For this review, take the finished solid that the model builds, in its own axes (mm). A direction names the side the tool comes from. Coordinates: 2 decimals unless noted, no trailing zeros. Order: outer loops, then holes, each group sorted by start corner. A loop starts at its lowest first (then second) coordinate and runs counter-clockwise, first axis right, second up. Notation, with made-up numbers: (-19, 10) -> (27, 10) arc R14 cw to (27, 28) -> close; hole circle Ø10 at (-24, -13). An arc over 180 degrees is marked (long way). Return JSON: item names as keys, results as strings. Group by question number.
Item 1: For line 1 along Y through (x, z) = (-13, 1); line 2 along Z through (x, y) = (29.5, 35); line 3 along X through (y, z) = (-1, 6), list the stretches that pass through material, from the lowest coordinate up.
Item 2: Take a section at A-A (y = 5). Write out the cut boundary in (x, z).
Item 3: Insertion check: pin 1 (12 mm diameter, centred on x = 0.5, y = 10.5, fed in from -Z); pin 2 (3 mm diameter, centred on x = 31.5, y = 80.5, fed in from +Z); pin 3 (3.5 mm diameter, centred on x = -36.93, y = 56.31, fed in from -Z); pin 4 (12 mm diameter, centred on y = -19.5, z = 9.5, fed in from -X). Each pin has a flat end and moves straight along its axis. Give the tip position at first contact, or say it passes through.
Item 4: Draft analysis for pull direction Z (two halves, no side actions). For faces 1 (the flat face through (0.57, -7.61, 11.68)), 2 (the flat face through (-10, -10, 4)), 3 (the cylindrical face through (0.567, -19.206, 5.344)), 4 (the cylindrical face through (-20.316, -19.206, 5.344)), state which applies: +Z half, -Z half, draft (parallel to the pull), parting line (faces both ways), or undercut.
Item 5: Take a section at B-B (x = 12.5). Write out the cut boundary in (y, z), then the cut area to 3 significant figures.
Item 6: Take a section at C-C (x = -6). Write out the cut boundary in (y, z).
Item 7: Take a section at D-D (z = -2.5). Write out the cut boundary in (x, y), then the cut area to 3 significant figures.
Item 8: Machinability: for faces 5 (the flat face through (10, -10, 4)), 6 (the flat face through (25, -16, 4)), 7 (the flat face through (20.183, -8.199, -3.475)), 8 (the flat face through (-20.316, -8.199, -3.475)), which of the approach directions +Z, -Z, +X, -X, +Y, -Y give a long, thin tool a straight path to every point of the face, cutting with its end or side? Answer none if there is none.
```python
from build123d import *

# Parameters (mm, degrees)
SKETCH_1_R                  = 2
SKETCH_1_R_2                = 23
EXTRUDE_1_DEPTH             = 8
SKETCH_2_R                  = 2.5
EXTRUDE_2_DEPTH             = 9.5
EXTRUDE_START               = -9.5
SKETCH_4_R                  = 2.5
EXTRUDE_4_DEPTH             = 9.5
SKETCH_6_R                  = 12.5
SKETCH_6_R_2                = 2.5
EXTRUDE_1_2_DEPTH           = 4.75
RIB_1_REACH                 = 123.764
SKETCH_7_WALL_W             = 264.861352648
SKETCH_7_WALL_H             = 9.5
EXTRUDE_5_DEPTH             = 9.5
EXTRUDE_6_DEPTH             = 9.5
CUT_EXTRUDE_3_REACH         = 110.864
SKETCH_20_R                 = 4
EXTRUDE_7_REACH             = 111.081
EXTRUDE_7_DIRECTION_2_REACH = 111.081
RIB_2_REACH                 = 123.764
SKETCH_14_WALL_W            = 263.59041227
SKETCH_14_WALL_H            = 9.5
RIB_3_REACH                 = 111.081
SKETCH_26_WALL_W            = 238.931348054
SKETCH_26_WALL_H            = 9.5


with BuildPart() as part:
    # 草图1 → Extrude 1 (new body)
    with BuildSketch(Plane.XY):
        with BuildLine():
            Line((-25, -10), (25, -10))
            Line((25, -10), (25, 10))
            ThreePointArc((25, 10), (0, 96.799497484), (-25, 10))
            Line((-25, 10), (-25, -10))
        make_face()
        with Locations((24.104535363, 78.526164101)):
            Circle(SKETCH_1_R, mode=Mode.SUBTRACT)
        with Locations((36.930290738, 56.311304147)):
            Circle(SKETCH_1_R, mode=Mode.SUBTRACT)
        with Locations((32.475952642, 31.049497484)):
            Circle(SKETCH_1_R, mode=Mode.SUBTRACT)
        with Locations((12.825755375, 14.561024205)):
            Circle(SKETCH_1_R, mode=Mode.SUBTRACT)
        with Locations((-12.825755375, 14.561024205)):
            Circle(SKETCH_1_R, mode=Mode.SUBTRACT)
        with Locations((-32.475952642, 31.049497484)):
            Circle(SKETCH_1_R, mode=Mode.SUBTRACT)
        with Locations((-36.930290738, 56.311304147)):
            Circle(SKETCH_1_R, mode=Mode.SUBTRACT)
        with Locations((-24.104535363, 78.526164101)):
            Circle(SKETCH_1_R, mode=Mode.SUBTRACT)
        with Locations((0, 87.299497484)):
            Circle(SKETCH_1_R, mode=Mode.SUBTRACT)
        with Locations((12.5, -5)):
            Circle(SKETCH_1_R, mode=Mode.SUBTRACT)
        with Locations(Location((-12.5, -5, 0), (0, 0, 180))):
            Circle(SKETCH_1_R, mode=Mode.SUBTRACT)
        with Locations((12.5, 5)):
            Circle(SKETCH_1_R, mode=Mode.SUBTRACT)
        with Locations(Location((-12.5, 5, 0), (0, 0, 180))):
            Circle(SKETCH_1_R, mode=Mode.SUBTRACT)
        with Locations((0, 49.799497484)):
            Circle(SKETCH_1_R_2, mode=Mode.SUBTRACT)
    extrude(amount=EXTRUDE_1_DEPTH)

    # 草图2 → 凸台-拉伸2 (add)
    with BuildSketch(Plane.ZY.offset(25)):
        with BuildLine():
            ThreePointArc((0, -10), (4, -33.313708499), (8, -10))
            Line((8, -10), (0, -10))
        make_face()
        with Locations((4, -21.313708499)):
            Circle(SKETCH_2_R, mode=Mode.SUBTRACT)
    extrude(amount=-EXTRUDE_2_DEPTH)

    # 草图4 → 凸台-拉伸4 (add)
    with BuildSketch(Plane(origin=(25, 0, 0), x_dir=(0, 0, -1), z_dir=(1, 0, 0)).offset(EXTRUDE_START)):
        with BuildLine():
            Line((-8, -10), (0, -10))
            ThreePointArc((0, -10), (-4, -33.313708499), (-8, -10))
        make_face()
        with Locations(Location((-4, -21.313708499, 0), (0, 0, 180))):
            Circle(SKETCH_4_R, mode=Mode.SUBTRACT)
    extrude(amount=EXTRUDE_4_DEPTH)

    # 草图6 → Extrude 1 2 (add, symmetric)
    with BuildSketch(Plane.ZY.offset(-0.5)):
        with Locations((4, -21.313708499)):
            Circle(SKETCH_6_R)
        with Locations((4, -21.313708499)):
            Circle(SKETCH_6_R_2, mode=Mode.SUBTRACT)
    extrude(amount=EXTRUDE_1_2_DEPTH, both=True)

    # 草图7 wall → 筋1 (add, up to next)
    with BuildSketch(Plane(origin=(-25, -8.913712594, 11.741206943), x_dir=(0, -0.922076341467, 0.387008036747), z_dir=(0, 0.387008036747, 0.922076341467)), mode=Mode.PRIVATE) as rib_1_sk1:
        with Locations((0, 4.75)):
            Rectangle(SKETCH_7_WALL_W, SKETCH_7_WALL_H)
    rib_1_tool1 = extrude(rib_1_sk1.sketch, amount=-RIB_1_REACH, mode=Mode.PRIVATE) - part.part
    add(rib_1_tool1.solids().sort_by_distance((-25, -8.913712594, 11.741206943))[0])

    # 草图12 → 凸台-拉伸5 (add)
    with BuildSketch(Plane(origin=(25, 0, 0), x_dir=(0, 0, -1), z_dir=(1, 0, 0))):
        Polygon((-8, 0), (-14.585289986, -15.537763557), (-9.647107703, -16.867490218), (-3.376423307, -1.94259218), align=None)
    extrude(amount=-EXTRUDE_5_DEPTH)

    # 草图15 → 凸台-拉伸6 (add)
    with BuildSketch(Plane.ZY.offset(25)):
        Polygon((0, 0), (-7.048639525, -16.631020739), (-1.081318286, -18.151978355), (5.605109172, -2.375584437), align=None)
    extrude(amount=-EXTRUDE_6_DEPTH)

    # 切除-拉伸3: up to this plane
    cut_extrude_3_end = Plane(origin=(-4.752183054, 0, 8), z_dir=(0, 0.390223979972796, 0.9207199603865396))
    # 草图20 → 切除-拉伸3 (cut, up to the surface)
    with BuildSketch(Plane.XY.offset(8), mode=Mode.PRIVATE) as cut_extrude_3_sk1:
        with Locations((-12.5, -5)):
            Circle(SKETCH_20_R)
    cut_extrude_3_tool1 = split(extrude(cut_extrude_3_sk1.sketch, amount=CUT_EXTRUDE_3_REACH, mode=Mode.PRIVATE), bisect_by=cut_extrude_3_end, keep=Keep.BOTH, mode=Mode.PRIVATE)
    add(cut_extrude_3_tool1.solids().sort_by_distance((-12.5, -5, 8))[0], mode=Mode.SUBTRACT)
    # 草图20 → 切除-拉伸3 (cut, up to the surface)
    with BuildSketch(Plane.XY.offset(8), mode=Mode.PRIVATE) as cut_extrude_3_sk2:
        with Locations((13.5, -5)):
            Circle(SKETCH_20_R)
    cut_extrude_3_tool2 = split(extrude(cut_extrude_3_sk2.sketch, amount=CUT_EXTRUDE_3_REACH, mode=Mode.PRIVATE), bisect_by=cut_extrude_3_end, keep=Keep.BOTH, mode=Mode.PRIVATE)
    add(cut_extrude_3_tool2.solids().sort_by_distance((13.5, -5, 8))[0], mode=Mode.SUBTRACT)

    # 凸台-拉伸7: up to this face of the body (flat: up to its plane)
    extrude_7_end = Plane(part.part.faces().sort_by_distance((-4.25, -9.735494608, -0.348936668))[0])
    # 草图23 → 凸台-拉伸7 (add, up to the picked face)
    with BuildSketch(Plane.ZY.offset(-0.5), mode=Mode.PRIVATE) as extrude_7_sk1:
        Polygon((3.246577314, -1.407985537), (-0.12612028, -0.27585848), (-7.368219852, -16.116249756), (-3.841621723, -16.91175555), align=None)
    extrude_7_tool1 = split(extrude(extrude_7_sk1.sketch, amount=EXTRUDE_7_REACH, mode=Mode.PRIVATE), bisect_by=extrude_7_end, keep=Keep.BOTH, mode=Mode.PRIVATE)
    add(extrude_7_tool1.solids().sort_by(Axis((0.5, -8.676237, -2.028521), (-1, 0, 0)))[0])

    # 凸台-拉伸7 direction 2: up to this face of the body (flat: up to its plane)
    extrude_7_direction_2_end = Plane(part.part.faces().sort_by_distance((5.25, -9.735494608, -0.348936668))[0])
    # 草图23 → 凸台-拉伸7 direction 2 (add, up to the picked face)
    with BuildSketch(Plane.ZY.offset(-0.5), mode=Mode.PRIVATE) as extrude_7_direction_2_sk1:
        Polygon((3.246577314, -1.407985537), (-0.12612028, -0.27585848), (-7.368219852, -16.116249756), (-3.841621723, -16.91175555), align=None)
    extrude_7_direction_2_tool1 = split(extrude(extrude_7_direction_2_sk1.sketch, amount=-EXTRUDE_7_DIRECTION_2_REACH, mode=Mode.PRIVATE), bisect_by=extrude_7_direction_2_end, keep=Keep.BOTH, mode=Mode.PRIVATE)
    add(extrude_7_direction_2_tool1.solids().sort_by(Axis((0.5, -8.676237, -2.028521), (1, 0, 0)))[0])

    # 草图14 wall → 筋2 (add, up to next)
    with BuildSketch(Plane(origin=(25, -8.31551037, -3.524319762), x_dir=(0, -0.920719960377, -0.390223979996), z_dir=(0, 0.390223979996, -0.920719960377)), mode=Mode.PRIVATE) as rib_2_sk1:
        with Locations((0, 4.75)):
            Rectangle(SKETCH_14_WALL_W, SKETCH_14_WALL_H)
    rib_2_tool1 = extrude(rib_2_sk1.sketch, amount=-RIB_2_REACH, mode=Mode.PRIVATE) - part.part
    add(rib_2_tool1.solids().sort_by_distance((25, -8.31551037, -3.524319762))[0])

    # 草图26 wall → 筋3 (add, up to next)
    with BuildSketch(Plane(origin=(0.5, -7.730285811, 11.733990841), x_dir=(0, -0.917438534624, 0.397877537927), z_dir=(0, 0.397877537927, 0.917438534624)), mode=Mode.PRIVATE) as rib_3_sk1:
        Rectangle(SKETCH_26_WALL_W, SKETCH_26_WALL_H)
    rib_3_tool1 = extrude(rib_3_sk1.sketch, amount=-RIB_3_REACH, mode=Mode.PRIVATE) - part.part
    add(rib_3_tool1.solids().sort_by_distance((0.5, -7.730285811, 11.733990841))[0])


solid = part.part
```
Findings below:
{
 "1": {"line 1": "y = -10 to -6.94, -3.06 to 3.06, 6.94 to 12.57, 16.55 to 30.83, 68.77 to 94.97", "line 2": "z = 0 to 8", "line 3": "x = -25 to 25"},
 "2": {"outline": "(-25, 0) -> (-14.5, 0) -> (-14.5, 8) -> (-25, 8) -> close; (-10.5, 0) -> (10.5, 0) -> (10.5, 8) -> (-10.5, 8) -> close; (14.5, 0) -> (25, 0) -> (25, 8) -> (14.5, 8) -> close"},
 "3": {"pin 1": "stops at z = 0", "pin 2": "stops at z = 8", "pin 3": "passes through", "pin 4": "stops at x = -25"},
 "4": {"face 1": "+Z half", "face 2": "draft", "face 3": "undercut", "face 4": "undercut"},
 "5": {"outline": "(-10, 0) -> (-7, 0) -> (-7, 8) -> (-10, 8) -> close; (-3, 0) -> (3, 0) -> (3, 8) -> (-3, 8) -> close; (7, 0) -> (12.59, 0) -> (12.59, 8) -> (7, 8) -> close; (16.53, 0) -> (30.49, 0) -> (30.49, 8) -> (16.53, 8) -> close; (69.11, 0) -> (95.11, 0) -> (95.11, 8) -> (69.11, 8) -> close", "area": "436 mm2"},
 "6": {"outline": "(-10, 0) -> (27.6, 0) -> (27.6, 8) -> (-10, 8) -> close; (72, 0) -> (96.41, 0) -> (96.41, 8) -> (72, 8) -> close"},
 "7": {"outline": "(-25, -31.4) -> (-15.5, -31.4) -> (-15.5, -5.9) -> (-25, -5.9) -> close; (-4.25, -31.99) -> (5.25, -31.99) -> (5.25, -5.47) -> (-4.25, -5.47) -> close; (15.5, -31.4) -> (25, -31.4) -> (25, -5.9) -> (15.5, -5.9) -> close", "area": "737 mm2"},
 "8": {"face 5": "+Z, -Z, -Y", "face 6": "+Z, -Z, +X, -Y", "face 7": "-Z, +X, +Y", "face 8": "-Z, -X, +Y"}
}
